Can you work these out from the model? Positions are in its coordinate system, mm. Face numbers are marked on the shaded views. A direction names the side the tool comes from. Coordinates: 2 decimals unless noted, no trailing zeros. Write each loop counter-clockwise with the first axis right and the second up, starting at its lowest first coordinate (ties: lowest second). Pieces come first, ordered by that corner, then holes. Notation, with made-up numbers: M 12.25,-40 L 51.25,-40 A25 cw 51.25,-6 Z; hole C 21.25,31.25 d1. An arc over 180 degrees is marked long. Answer as a JSON object with one key per item and string values. Group by question number.
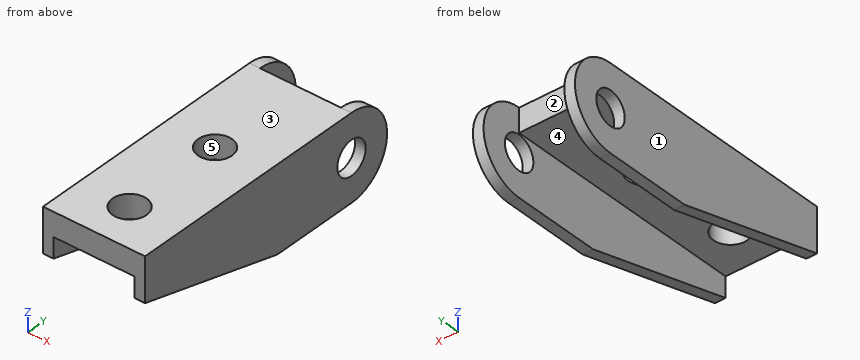
Autodesk Inventor part; units mm, degrees
ref_plane "YZ Plane" through (0, 0, 0) normal (1, 0, 0) x (0, 1, 0)
ref_plane "XZ Plane" through (0, 0, 0) normal (0, 1, 0) x (-1, 0, 0)
ref_plane "XY Plane" through (0, 0, 0) normal (0, 0, 1) x (1, 0, 0)
sketch "Эскиз1" plane through (0, 0, 0) normal (1, 0, 0) x (0, 1, 0)
  circle A0 centre (0, 0) radius 2
  arc A1 (-4.49, 2.2) -> (0, 5) centre (0, 0) ccw
  line L0 (0, 5) -> (-29, 5)
  line L1 (-29, 5) -> (-29, -0.2)
  line L2 (-29, -0.2) -> (-10.4, -5)
  line L3 (-10.4, -5) -> (0, -5)
  line L4 (-4.49, 2.2) -> (-29, 2.2)
  line L5 (-4.49, 5) -> (0, 5)
  line L6 (-4.49, 5) -> (-29, 5)
  line L7 (-10.4, -5) -> (0, -5)
  line L8 (-4.49, 2.2) -> (0, 2.2)
  line L9 (0, 2.2) -> (0, 5)
  line L10 (0, 5) -> (-4.49, 5)
  dimension "d0" = 4
  dimension "d1" = 10
  dimension "d2" = 34
  dimension "d3" = 5.2
  dimension "d4" = 18.6
  dimension "d5" = 2.8
  dimension "d6" = 10
extrude "Выдавливание1" add sketch "Эскиз1" along normal mid plane 12
extrude "Выдавливание2" cut sketch "Эскиз1" along normal mid plane 9.5 contours L8 L9 A1
extrude "Выдавливание3" cut sketch "Эскиз1" along normal mid plane 9.5 contours A1 L3 L2 L1 L4
sketch "Эскиз2" plane through (-6, -29, 5) normal (0, 0, 1) x (1, 0, 0)
  line L0 (6, 29) -> (6, 0) construction
  line L1 (0, 0) -> (12, 0) construction
  circle A0 centre (6, 5) radius 2
  circle A1 centre (6, 17) radius 2
  dimension "d13" = 4
  dimension "d14" = 4
  dimension "d15" = 12
  dimension "d16" = 5
extrude "Выдавливание4" cut sketch "Эскиз2" against normal blind 9.5
properties part number "крепленеи кабеля"
Q1. On a 3-axis mill with a long thin cutter (end or side, diameter ignored), from which of +Z, -Z, +X, -X, +Y, -Y can I reach the whole of each face in a straight line? I mean the marked faces 4 and 5. Say none if no direction works.
Q2. If we section it at B-B on z = -3: List the corners of the cut face in (x, y) for me, and give its area (3 significant figures).
Q3. If we section it at A-A on x = 0: List the corners of the cut face in (y, z) for me.
Q4. We'd pull the mould along X, two halves only. Please class the marked faces 1, 2 and 3: pulls with the +X half, pulls with the -X half, needs draft (parallel to the pull), parting line crosses it, or undercut.
Q5. If we section it at D-D on z = 1.5: List the corners of the cut face in (x, y) for me.
Q6. Will these pins go through, and if not, where does the flat tip stop? pin 1 (2.5 mm diameter, centred on x = 0, y = -12, fed in from +Z); pin 2 (1.5 mm diameter, centred on x = -2, y = -23, fed in from -Z); pin 3 (4 mm diameter, centred on x = -2.5, z = 2, fed in from +Y); pin 4 (1 mm diameter, centred on x = -5, z = 3.5, fed in from +Y).
Q7. If we section it at C-C on y = 0.5: List the corners of the cut face in (x, z) for me.
Q8. Please list where these lines run through material, in increasing order: L1, parallel to X at y = 3, z = 3; L2, parallel to Z at x = 5.1, y = 0; L3, parallel to Y at x = 0, z = 3.05.
Reply:
{
 "1": {"face 4": "-Z, +Y, -Y", "face 5": "+Z, -Z"},
 "2": {"outline": "M -6,-18.15 L -4.75,-18.15 L -4.75,4 L -6,4 Z; M 4.75,-18.15 L 6,-18.15 L 6,4 L 4.75,4 Z", "area": "55.4 mm^2"},
 "3": {"outline": "M -29,2.2 L -26,2.2 L -26,5 L -29,5 Z; M -22,2.2 L -14,2.2 L -14,5 L -22,5 Z; M -10,2.2 L 0,2.2 L 0,5 L -10,5 Z"},
 "4": {"face 1": "pulls with the -X half", "face 2": "undercut", "face 3": "needs draft"},
 "5": {"outline": "M -6,-29 L -4.75,-29 L -4.75,-1.32 L -6,-1.32 Z; M -6,1.32 L -4.75,1.32 L -4.75,4.77 L -6,4.77 Z; M 4.75,-29 L 6,-29 L 6,-1.32 L 4.75,-1.32 Z; M 4.75,1.32 L 6,1.32 L 6,4.77 L 4.75,4.77 Z"},
 "6": {"pin 1": "through", "pin 2": "z = 2.2", "pin 3": "y = 0", "pin 4": "y = 4"},
 "7": {"outline": "M -6,-4.97 L -4.75,-4.97 L -4.75,-1.94 L -6,-1.94 Z; M -6,1.94 L -4.75,1.94 L -4.75,4.97 L -6,4.97 Z; M 4.75,-4.97 L 6,-4.97 L 6,-1.94 L 4.75,-1.94 Z; M 4.75,1.94 L 6,1.94 L 6,4.97 L 4.75,4.97 Z"},
 "8": {"L1": "-6 to -4.75, 4.75 to 6", "L2": "-5 to -2, 2 to 5", "L3": "-29 to -26, -22 to -14, -10 to 0"}
}
